Could you check a few things on this model? Use its own coordinates, in mm. Face numbers are marked on the shaded views. A direction names the side the tool comes from. Give positions to 0.01 mm unless a question says otherwise; leave off trailing zeros. Write each loop counter-clockwise with the first axis right and the second up, starting at its lowest first coordinate (ties: lowest second). Pieces come first, ordered by that corner, then holes. Notation, with made-up numbers: (-0.75, -18.5) -> (35.25, -18.5) arc R14 ccw to (35.25, -11.5) -> close; hole circle Ø11 at (-21, 23). An arc over 180 degrees is marked (long way). One line per question, with ' | ' between items.
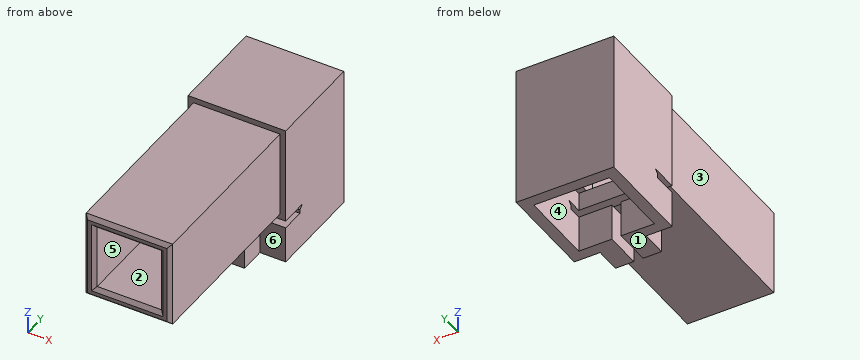
from build123d import *

# Parameters (mm, degrees)
PAD_DEPTH       = 10
PAD001_DEPTH    = 2
CHAMFER_SIZE    = 1
SKETCH002_W     = 26.5
SKETCH002_H     = 26.5
PAD002_DEPTH    = 26.5
SKETCH003_W     = 16.5
SKETCH003_H     = 16.5
POCKET_DEPTH    = 20
SKETCH004_W     = 20.5
SKETCH004_H     = 20.5
POCKET001_DEPTH = 5
SKETCH005_W     = 23.45
SKETCH005_H     = 23.45
SKETCH005_W_2   = 17.45
SKETCH005_H_2   = 17.45
PAD003_DEPTH    = 50
CHAMFER001_SIZE = 1


with BuildPart() as part:
    # Sketch → Pad (new body)
    with BuildSketch(Plane.XY):
        Polygon((6.25, -20.25), (6.25, -13.25), (13.25, -13.25), (13.25, 13.25), (-13.25, 13.25), (-13.25, -13.25), (-6.25, -13.25), (-6.25, -20.25), (-1.25, -20.25), (-1.25, -10.25), (-10.25, -10.25), (-10.25, 10.25), (10.25, 10.25), (10.25, -10.25), (1.25, -10.25), (1.25, -20.25), align=None)
    extrude(amount=PAD_DEPTH)

    # Sketch001 (on Face18 of Pad) → Pad001 (join)
    with BuildSketch(Plane.XY.offset(10)):
        Polygon((-10.25, -6.75), (-13.25, -6.75), (-13.25, 13.25), (13.25, 13.25), (13.25, -6.75), (10.25, -6.75), (10.25, 10.25), (-10.25, 10.25), align=None)
    extrude(amount=PAD001_DEPTH)

    # Chamfer
    chamfer_edges = [part.edges().sort_by_distance(p)[0] for p in [
        (-11.75, -6.75, 12),
        (11.75, -6.75, 12),
    ]]
    chamfer(chamfer_edges, length=CHAMFER_SIZE)

    # Sketch002 (on Face7 of Chamfer) → Pad002 (join)
    with BuildSketch(Plane.XY.offset(12)):
        Rectangle(SKETCH002_W, SKETCH002_H)
    extrude(amount=PAD002_DEPTH)

    # Sketch003 (on Face20 of Pad002) → Pocket (cut)
    with BuildSketch(Plane.XZ.offset(13.25)):
        with Locations((0, 25.25)):
            Rectangle(SKETCH003_W, SKETCH003_H)
    extrude(amount=-POCKET_DEPTH, mode=Mode.SUBTRACT)

    # Sketch004 (on Face9 of Pocket) → Pocket001 (cut)
    with BuildSketch(Plane(origin=(0, 0, 12), x_dir=(1, 0, 0), z_dir=(0, 0, -1))):
        Rectangle(SKETCH004_W, SKETCH004_H)
    extrude(amount=-POCKET001_DEPTH, mode=Mode.SUBTRACT)

    # Sketch005 (on Face21 of Pocket001) → Pad003 (join)
    with BuildSketch(Plane.XZ.offset(13.25)):
        with Locations((0, 25.25)):
            Rectangle(SKETCH005_W, SKETCH005_H)
        with Locations((0, 25.25)):
            Rectangle(SKETCH005_W_2, SKETCH005_H_2, mode=Mode.SUBTRACT)
    extrude(amount=PAD003_DEPTH)

    # Chamfer001
    chamfer001_edges = [part.edges().sort_by_distance(p)[0] for p in [
        (0, -63.25, 36.975),
        (11.725, -63.25, 25.25),
        (0, -63.25, 13.525),
        (-11.725, -63.25, 25.25),
        (0, -63.25, 33.975),
        (8.725, -63.25, 25.25),
        (0, -63.25, 16.525),
        (-8.725, -63.25, 25.25),
    ]]
    chamfer(chamfer001_edges, length=CHAMFER001_SIZE)


solid = part.part
Q1. If we mould it in two halves opening along Z, with no side actions, what happens to the marked faces 1, 2 and 3? For each: +Z half, -Z half, draft (parallel to the pull), parting line (faces both ways), or undercut.
Answer below:
face 1: -Z half | face 2: undercut | face 3: draft
Q2. Imagine slicing it at B-B on x = 4.25. Please give me the cut outline in (y, z) (3 decimals).
Answer below:
outline: (-63.25, 14.525) -> (-62.25, 13.525) -> (-13.25, 13.525) -> (-13.25, 12) -> (-10.25, 12) -> (-10.25, 17) -> (-13.25, 17) -> (-13.25, 16.525) -> (-62.25, 16.525) -> (-63.25, 15.525) -> close; (-63.25, 34.975) -> (-62.25, 33.975) -> (-13.25, 33.975) -> (-13.25, 33.5) -> (6.75, 33.5) -> (6.75, 17) -> (10.25, 17) -> (10.25, 0) -> (13.25, 0) -> (13.25, 38.5) -> (-13.25, 38.5) -> (-13.25, 36.975) -> (-62.25, 36.975) -> (-63.25, 35.975) -> close; (-20.25, 0) -> (-10.25, 0) -> (-10.25, 10) -> (-20.25, 10) -> close
Q3. On a 3-axis mill with a long thin cutter (end or side, diameter ignored), from which of +Z, -Z, +X, -X, +Y, -Y can I reach the whole of each face in a straight line? I mean the marked faces 4, 5 and 6. Say none if no direction works.
Answer below:
face 4: -Z | face 5: -Y | face 6: -Z, +X, -Y
Q4. Will these pins go through, and if not, where does the flat tip stop? pin 1 (3 mm diameter, centred on x = -2.5, y = -29, fed in from -Z) (3 decimals); pin 2 (7 mm diameter, centred on y = -28.5, z = 28, fed in from +X) (3 decimals); pin 3 (11.5 mm diameter, centred on y = -27, z = 27, fed in from -X) (3 decimals).
Answer below:
pin 1: stops at z = 13.525 | pin 2: stops at x = 11.725 | pin 3: stops at x = -11.725
Q5. Imagine slicing it at A-A on y = -14.5. Please give me the cut outline in (x, z) (3 decimals).
Answer below:
outline: (-11.725, 13.525) -> (11.725, 13.525) -> (11.725, 36.975) -> (-11.725, 36.975) -> close; (-6.25, 0) -> (-1.25, 0) -> (-1.25, 10) -> (-6.25, 10) -> close; (1.25, 0) -> (6.25, 0) -> (6.25, 10) -> (1.25, 10) -> close; hole (-8.725, 16.525) -> (8.725, 16.525) -> (8.725, 33.975) -> (-8.725, 33.975) -> close
Q6. Imagine slicing it at D-D on y = -47. Please give me the cut outline in (x, z) (3 decimals), and give its area (3 significant figures).
Answer below:
outline: (-11.725, 13.525) -> (11.725, 13.525) -> (11.725, 36.975) -> (-11.725, 36.975) -> close; hole (-8.725, 16.525) -> (8.725, 16.525) -> (8.725, 33.975) -> (-8.725, 33.975) -> close | area: 245 mm^2
Q7. If I drill on line 1 along X through (y, z) = (-10, 19); line 2 along Z through (x, y) = (-8.25, -45) (3 decimals); line 3 along Y through (x, z) = (-9, 15.5), over which ranges is the centre line in solid material (lowest first)?
Answer below:
line 1: x = -13.25 to -8.25, 8.25 to 13.25 | line 2: z = 13.525 to 16.525, 33.975 to 36.975 | line 3: y = -63.25 to -10.25, 10.25 to 13.25
Q8. Imagine slicing it at C-C on x = 0.5. Please give me the cut outline in (y, z) (3 decimals), and give its area (3 significant figures).
Answer below:
outline: (-63.25, 14.525) -> (-62.25, 13.525) -> (-13.25, 13.525) -> (-13.25, 12) -> (-10.25, 12) -> (-10.25, 17) -> (-13.25, 17) -> (-13.25, 16.525) -> (-62.25, 16.525) -> (-63.25, 15.525) -> close; (-63.25, 34.975) -> (-62.25, 33.975) -> (-13.25, 33.975) -> (-13.25, 33.5) -> (6.75, 33.5) -> (6.75, 17) -> (10.25, 17) -> (10.25, 0) -> (13.25, 0) -> (13.25, 38.5) -> (-13.25, 38.5) -> (-13.25, 36.975) -> (-62.25, 36.975) -> (-63.25, 35.975) -> close | area: 604 mm^2
